Here's how the part is built. I have some questions about the finished solid (model axes, mm). Give positions to 0.01 mm unless a question says otherwise; leave off trailing zeros. Loops run counter-clockwise (first coordinate to the right, second up) from the corner with the lowest first, then second, coordinate; pieces in that order, holes last. Notation, with made-up numbers: (89, 13) -> (121, 13) arc R13 ccw to (121, 23) -> close; hole circle Ø9 at (42.5, 77). An arc over 180 degrees is marked (long way). Answer in a Markdown table with one row per item. Add a question column.
Item 1: For P1, Ø2.5, axis at x = -44.54, y = -14.05, coming from the +Z side, with a flat end and sliding along its axis, tell me the tip position at first contact or that it passes through.
Item 2: If I drill on line 1 (Y direction, x = -47, z = 3.75); line 2 (X direction, y = -4.05, z = 2.25); line 3 (X direction, y = -14.05, z = 3.9), over which ranges is the centre line in solid material (lowest first)?
Item 3: If we section it at A-A (y = 15.95): Write out the boundary of the cut face in (x, z), then the cut area to 3 significant figures.
Item 4: If we section it at B-B (x = -34): Write out the boundary of the cut face in (y, z).
Item 5: If we section it at C-C (z = 4.35): Give the number of separate pieces and of enclosed holes in the cut face, then the cut area to 3 significant figures.
Item 6: We'd pull the mould along X, two halves only. Please class faces 1 (the face through (-48.5, -4, 2.5)), 2 (the face through (-53, -2, 3)), 3 (the face through (-38, 20.95, 3)): released by +X, released by -X, zero draft, split by the parting line, or undercut.
```python
from build123d import *

# Parameters (mm, degrees)
SKETCH_1_W               = 30
SKETCH_1_H               = 45
EXTRUDE_1_DEPTH          = 5.15
CUT_EXTRUDE_1_DEPTH      = 59.428802829
CUT_EXTRUDE_1_DEPTH_BACK = 59.428802829
SKETCH_2_R               = 1.5
CUT_EXTRUDE_2_DEPTH      = 59.428802829
CUT_EXTRUDE_2_DEPTH_BACK = 59.428802829
SKETCH_3_R               = 1.5
SKETCH_3_R_2             = 1.513831086


with BuildPart() as part:
    # 草图1 → 凸台-拉伸1 (new body)
    with BuildSketch(Plane.XY):
        with Locations((-38, -1.55)):
            Rectangle(SKETCH_1_W, SKETCH_1_H)
    extrude(amount=EXTRUDE_1_DEPTH)

    # 草图2 → 切除-拉伸1 (cut, two sides: drawn at the far end of the back side and taken through both)
    with BuildSketch(Plane.XY.offset(5.15).offset(-CUT_EXTRUDE_1_DEPTH_BACK)):
        with Locations((-34, 15.95)):
            Circle(SKETCH_2_R)
        with Locations((-47, 15.95)):
            Circle(SKETCH_2_R)
        with Locations((-34, -4.05)):
            Circle(SKETCH_2_R)
        with Locations((-47, -4.05)):
            Circle(SKETCH_2_R)
    extrude(amount=CUT_EXTRUDE_1_DEPTH + CUT_EXTRUDE_1_DEPTH_BACK, mode=Mode.SUBTRACT)

    # 草图3 → 切除-拉伸2 (cut, two sides: drawn at the far end of the back side and taken through both)
    with BuildSketch(Plane.XY.offset(5.15).offset(-CUT_EXTRUDE_2_DEPTH_BACK)):
        with Locations((-44.544155877, -14.05)):
            Circle(SKETCH_3_R)
        with Locations((-37.544155877, -14.05)):
            Circle(SKETCH_3_R)
        with Locations((-44.544155877, 1.95)):
            Circle(SKETCH_3_R_2)
        with Locations((-37.544155877, 1.95)):
            Circle(SKETCH_3_R)
    extrude(amount=CUT_EXTRUDE_2_DEPTH + CUT_EXTRUDE_2_DEPTH_BACK, mode=Mode.SUBTRACT)


solid = part.part
```
Recorded:
| question | item | result |
|---|---|---|
| 1 | P1 | passes through |
| 2 | line 1 | y = -24.05 to -5.55, -2.55 to 14.45, 17.45 to 20.95 |
| 2 | line 2 | x = -53 to -48.5, -45.5 to -35.5, -32.5 to -23 |
| 2 | line 3 | x = -53 to -46.04, -43.04 to -39.04, -36.04 to -23 |
| 3 | outline | (-53, 0) -> (-48.5, 0) -> (-48.5, 5.15) -> (-53, 5.15) -> close; (-45.5, 0) -> (-35.5, 0) -> (-35.5, 5.15) -> (-45.5, 5.15) -> close; (-32.5, 0) -> (-23, 0) -> (-23, 5.15) -> (-32.5, 5.15) -> close |
| 3 | area | 124 mm^2 |
| 4 | outline | (-24.05, 0) -> (-5.55, 0) -> (-5.55, 5.15) -> (-24.05, 5.15) -> close; (-2.55, 0) -> (14.45, 0) -> (14.45, 5.15) -> (-2.55, 5.15) -> close; (17.45, 0) -> (20.95, 0) -> (20.95, 5.15) -> (17.45, 5.15) -> close |
| 5 | separate pieces | 1 |
| 5 | enclosed holes | 8 |
| 5 | area | 1,290 mm^2 |
| 6 | face 1 | undercut |
| 6 | face 2 | released by -X |
| 6 | face 3 | zero draft |
